Check sheet for the modelled part. Datum: model origin and axes. Units: mm. A direction names the side the tool comes from. Round coordinates to 2 decimals unless told otherwise and drop trailing zeros. Loops run counter-clockwise (first coordinate to the right, second up) from the corner with the lowest first, then second, coordinate; pieces in that order, holes last. Notation, with made-up numbers: M 32.25,13 L 59.25,13 A16 ccw 59.25,18 Z; hole C 31.25,68.5 d4. An arc over 180 degrees is marked long. One line per question, with ' | ' between items. Start each with the question number.
(1) Section check C-C (y = 39). Record the boundary of the cut face in (x, z), and give its area (3 significant figures).
(2) Draft check along Z on faces 5 (the face through (-16, -40, -47.709)), 6 (the face through (-15, 25, 0)), 7 (the face through (-30, 25, -15)), 8 (the face through (-16, -15, -45)). Enter one of: +Z half, -Z half, draft (parallel to the pull), parting line (faces both ways), or undercut.
(3) Tool access check on faces 1 (the face through (-27, 24, -15)), 2 (the face through (-15, 25, -30)), 3 (the face through (-14, -42, 25)), 4 (the face through (-14.58, -12.62, -37.87)). Record the directions out of +Z, -Z, +X, -X, +Y, -Y that give a thin tool (end or side, any length) a straight path to the whole face; none if there is none.
(4) Section check D-D (y = -50.5). Record the boundary of the cut face in (x, z), and give its area (3 significant figures).
(5) Thickness scan on probe 1 along Z at (x, y) = (-19, -33); probe 2 along Z at (x, y) = (-18, 22.5). Record the ranges inside material, lowest first. Write a range as [from, to].
(6) Go/stop test with flat-tipped pins: P1, Ø12, axis at x = -15.5, y = 32.5, coming from the -Z side; P2, Ø1, axis at y = 25, z = -6, coming from the +X side; P3, Ø5, axis at x = 11, z = -37.5, coming from the +Y side. Record where each tip stops, or that it passes through.
Autodesk Inventor part; units mm, degrees
ref_plane "YZ Plane" through (0, 0, 0) normal (1, 0, 0) x (0, 1, 0)
ref_plane "XZ Plane" through (0, 0, 0) normal (0, 1, 0) x (-1, 0, 0)
ref_plane "XY Plane" through (0, 0, 0) normal (0, 0, 1) x (1, 0, 0)
sketch "Boceto1" plane through (0, 0, 0) normal (0, 1, 0) x (-1, 0, 0)
  line L0 (0, 0) -> (30, 0)
  line L1 (30, 0) -> (30, -30)
  line L2 (30, -30) -> (0, -30)
  line L3 (0, -30) -> (0, 0)
  dimension "d0" = 30
  dimension "d1" = 30
extrude "Extrusión1" add sketch "Boceto1" along normal blind 50
sketch "Boceto2" plane through (0, 50, 0) normal (0, 1, 0) x (1, 0, 0)
  line L0 (-30, 0) -> (0, 0)
  line L1 (0, 0) -> (-3, 0)
  line L2 (-3, 0) -> (-6, 0)
  line L3 (-3, 0) -> (-3, 3)
  line L4 (-30, 30) -> (-30, 0)
  line L5 (-30, 30) -> (-27, 30)
  line L6 (0, 30) -> (-30, 30)
  line L7 (-27, 30) -> (-30, 30)
  line L8 (-27, 30) -> (-27, 27)
  line L9 (-3, 3) -> (-27, 3)
  line L10 (-27, 3) -> (-27, 27)
  line L11 (-27, 27) -> (-3, 27)
  line L12 (-3, 27) -> (-3, 3)
  dimension "d4" = 3
  dimension "d6" = 3
  dimension "d7" = 3
  dimension "d8" = 3
  dimension "d9" = 3
extrude "Extrusión2" cut sketch "Boceto2" against normal blind 184.25 contours L9 L10 L11 L12
sketch "Boceto3" plane through (0, 0, 0) normal (1, 0, 0) x (0, 0, -1)
  point P0 (0, 0)
sketch "Boceto4" plane through (0, 0, 0) normal (0, -1, 0) x (1, 0, 0)
  line L0 (25, 25) -> (-55, 25)
  line L1 (-55, 25) -> (-55, -55)
  line L2 (-55, -55) -> (25, -55)
  line L3 (25, -55) -> (25, 25)
  line L4 (25, -55) -> (25, -15)
  line L5 (25, -15) -> (-15, -15)
  line L6 (0, 0) -> (0, -30)
  line L7 (0, 0) -> (0, -15)
  line L8 (0, -15) -> (-15, -15)
  dimension "d12" = 80
  dimension "d13" = 80
  dimension "d14" = 40
  dimension "d15" = 40
  dimension "d16" = 15
  dimension "d17" = 15
extrude "Extrusión3" add sketch "Boceto4" along normal blind 60
chamfer "Chaflán1" distance 25 angle 45 1 edges at (-55, 0, -15)
chamfer "Chaflán2" distance 25 angle 45 1 edges at (-2.5003, 0, 25)
chamfer "Chaflán3" distance 25 angle 45 1 edges at (-2.5003, 0, -55)
chamfer "Chaflán4" distance 25 angle 45 1 edges at (25, 0, -15)
sketch "Boceto6" plane through (0, -60, 0) normal (0, -1, 0) x (1, 0, 0)
  line L0 (0, 0) -> (25, 25)
  line L1 (-55, -55) -> (-30, -30)
  line L2 (15.6406, 15.6406) -> (-47.7087, 15.6406)
  line L3 (-47.7087, 15.6406) -> (-47.7087, -47.7087)
  line L4 (-47.7087, -47.7087) -> (15.6406, -47.7087)
  line L5 (15.6406, -47.7087) -> (15.6406, 15.6406)
extrude "Extrusión5" cut sketch "Boceto6" against normal blind 40.25
sketch "Boceto7" plane through (0, 0, 0) normal (0, 1, 0) x (1, 0, 0)
  line L0 (-3, 27) -> (-27, 27)
  line L1 (-3, 3) -> (-3, 27)
  line L2 (-27, 27) -> (-3, 27)
  line L3 (-3, 27) -> (-3, 3)
  line L4 (-3, 3) -> (-27, 3)
  line L5 (-27, 3) -> (-27, 27)
  point P0 (0, 0)
extrude "Extrusión6" cut sketch "Boceto7" against normal blind 184.25
chamfer "Chaflán5" distance 18 angle 45 4 edges at (-27, -19.75, -15) (-15, -19.75, -3) (-15, -19.75, -27) (-3, -19.75, -15)
properties part number "tolva"
The answers:
1) outline: M -30,-30 L 0,-30 L 0,0 L -30,0 Z; hole M -27,-27 L -3,-27 L -3,-3 L -27,-3 Z | area: 324 mm²
2) face 5: undercut | face 6: +Z half | face 7: draft | face 8: -Z half
3) face 1: +Y, -Y | face 2: -Z, +X, -X, +Y | face 3: +Z, +X, -X, +Y, -Y | face 4: -Y
4) outline: M -55,-55 L 25,-55 L 25,25 L -55,25 Z; hole M -47.71,-47.71 L 15.64,-47.71 L 15.64,15.64 L -47.71,15.64 Z | area: 2,390 mm²
5) probe 1: [-55, -47.71], [15.64, 25] | probe 2: [-30, -27], [-3, 0]
6) P1: z = -30 | P2: x = 0 | P3: y = -8.5
